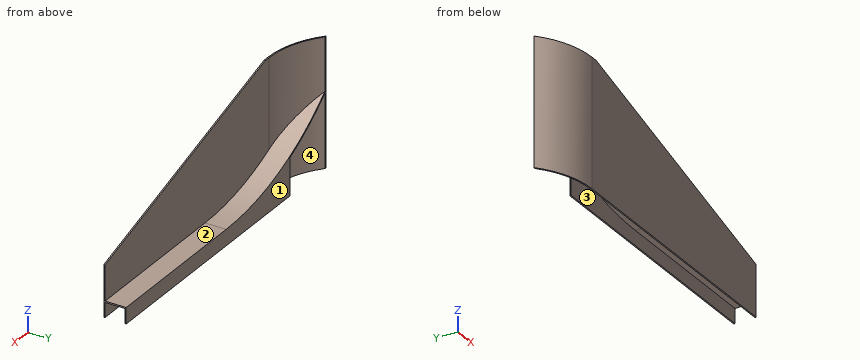
Autodesk Inventor part; units mm, degrees
ref_plane "YZ Plane" through (0, 0, 0) normal (1, 0, 0) x (0, 1, 0)
ref_plane "XZ Plane" through (0, 0, 0) normal (0, 1, 0) x (-1, 0, 0)
ref_plane "XY Plane" through (0, 0, 0) normal (0, 0, 1) x (1, 0, 0)
sketch "スケッチ1" plane through (0, 0, 0) normal (0, 1, 0) x (-1, 0, 0)
  line L0 (250, 100) -> (-250, 100)
  line L1 (-250, 100) -> (-250, -100)
  line L2 (-250, -100) -> (250, -100)
  line L3 (250, -100) -> (250, 100)
  point P0 (0, 0)
  dimension "d2" = 250
  dimension "d3" = 500
  dimension "d4" = 100
  dimension "d5" = 200
extrude "押し出し1" add sketch "スケッチ1" along normal blind 35
sketch "スケッチ2" plane through (-250, 0, 100) normal (0, 0, 1) x (1, 0, 0)
  line L0 (0, 35) -> (500, 35)
  line L1 (0, 0) -> (500, 0)
  arc A0 (0, 35) -> (90, 0) centre (90, 133.2143) ccw
  line L2 (0, 0) -> (0, 35)
  point P0 (250, 0)
  dimension "d8" = 90
extrude "押し出し2" cut sketch "スケッチ2" against normal through all
sketch "スケッチ5" plane through (-160, 0, 100) normal (0, 0, 1) x (1, 0, 0)
  arc A0 (-90, 35) -> (0, 0) centre (0, 133.2143) ccw
  line L0 (0, 0) -> (410, 0)
  arc A1 (-87.0123, 35) -> (0, 2) centre (0, 133.2143) ccw
  line L1 (0, 2) -> (54.4195, 2)
  line L2 (54.4195, 2) -> (410, 2)
  line L3 (-90, 35) -> (410, 35)
  line L4 (410, 0) -> (410, 35)
  point P0 (160, 0)
  point P1 (40, 35)
  dimension "d20" = 2
extrude "押し出し5" cut sketch "スケッチ5" against normal through all contours L3 L4 L2 L1 A1
sketch "スケッチ8" plane through (-160, 2, 100) normal (0, 1, 0) x (1, 0, 0)
  line L0 (410, 175) -> (160, 175)
  line L1 (410, 200) -> (410, 0)
  line L2 (0, 200) -> (410, 200)
  arc A0 (160, 175) -> (-90, 80) centre (160, -201.4474) ccw
  line L3 (-90, 200) -> (-90, 0)
  line L4 (-87.0123, 200) -> (0, 200)
  line L5 (-87.0123, 200) -> (-90, 200)
  line L6 (410, 177) -> (160, 177)
  arc A1 (160, 177) -> (-90, 82.6695) centre (160, -201.4474) ccw
  line L7 (410, 175) -> (410, 177)
  line L8 (410, 0) -> (410, 200)
  line L9 (-90, 82.6695) -> (-90, 80)
  point P0 (160, 100)
  dimension "d35" = 25
  dimension "d36" = 120
  dimension "d37" = 250
  dimension "d38" = 2
extrude "押し出し7" add sketch "スケッチ8" along normal up to surface (33 mm away) contours L0 A0 L3 A1 L6 L1
delete faces "面を削除1" heal yes whole lump no faces at (-239.2435, 9.8792, 10.8013) (-250, 24, 18.2203) (-242.947, 2, 13.2909) (-239.2361, 9.8796, 8.2094)
sketch "スケッチ9" plane through (0, 35, -75) normal (0, 1, 0) x (1, 0, 0)
  line L0 (250, 25) -> (250, 2)
  line L1 (0, 2) -> (250, 2)
  line L2 (250, 25) -> (250, 2)
  line L3 (-160, 25) -> (250, 25)
  line L4 (-160, -33.4861) -> (-160, 25)
  arc A0 (0, 2) -> (-160, -33.4861) centre (0, -376.4474) ccw
  point P0 (0, -75)
extrude "押し出し8" add sketch "スケッチ9" against normal blind 2
sketch "スケッチ10" plane through (-160, 2, 100) normal (0, 1, 0) x (1, 0, 0)
  line L0 (410, 175) -> (410, 0)
  line L1 (410, 0) -> (0, 0)
  line L2 (410, 0) -> (410, 200)
  line L3 (410, 120) -> (10, 0)
  line L4 (0, 0) -> (410, 0)
  point P0 (160, 100)
  dimension "d43" = 400
  dimension "d44" = 120
extrude "押し出し9" cut sketch "スケッチ10" against normal through all
properties part number "endplate_ver2"
Work out the finished part from the listing and answer in its coordinate system (mm). Face numbers are marked on the shaded views. A direction names the side the tool comes from. Coordinates: 2 decimals unless noted, no trailing zeros. Loops run counter-clockwise (first coordinate to the right, second up) from the corner with the lowest first, then second, coordinate; pieces in that order, holes last. Notation, with made-up numbers: M 11,16 L 28,16 A20 ccw 28,34 Z; hole C 10,-6.75 d1. An arc over 180 degrees is marked long. Use CSV: the item, a comma, the result in double quotes. Start each with the question number.
(1) Find section B-B, the plane y = 20. Give the vertices of the cut face in (x, z), then the cut area to 3 significant figures.
(2) Given pin 1 Ø2 at (y, z) = (27, 2) entering from -X; pin 2 Ø4 at (x, z) = (-164.5, -26) entering from +Y; pin 3 Ø8 at (x, y) = (-123, 29.5) entering from +Z, each flat-ended and moving along its own axis, determine where each tip first touches the part or whether it passes through.
(3) For the marked faces 1, 2, 3 and 4, determine the directions among +Z, -Z, +X, -X, +Y, -Y from which every point of the face is accessible in a straight line to the end or side of a thin tool.
(4) Find section D-D, the plane z = 30. Give the vertices of the cut face in (x, y).
(5) Find section A-A, the plane x = 138.5. Give the vertices of the cut face in (y, z), then the cut area to 3 significant figures.
(6) Consider line 1 (Y direction, x = 212, z = -87.5); line 2 (Y direction, x = -146, z = -30); line 3 (Z direction, x = 5, y = 13). Determine where each line is inside the solid, lowest interval first.
Recorded:
1,outline,"M -230.2,-100 L -226.33,-100 L -226.33,-1.86 A378.45 ccw 0,-77 L 250,-77 L 250,-75 L 0,-75 A376.45 cw -226.33,0.64 L -226.33,100 L -230.2,100 Z"
1,area,"1,760 mm^2"
2,pin 1,"stops at x = -241.71"
2,pin 2,"stops at y = 2.16"
2,pin 3,"stops at z = -52.93"
3,face 1,"+Z, -Z, +X, -X, +Y"
3,face 2,"+Z, +X, +Y"
3,face 3,"-Z"
3,face 4,"-Z, +Y"
4,outline,"M -250,35 A133.21 ccw -160,0 L 83.33,0 L 83.33,2 L -160,2 A131.21 cw -247.01,35 Z"
5,outline,"M 0,-100 L 2,-100 L 2,-77 L 33,-77 L 33,-100 L 35,-100 L 35,-75 L 2,-75 L 2,13.45 L 0,13.45 Z"
5,area,"339 mm^2"
6,line 1,"y = 0 to 2, 33 to 35"
6,line 2,"y = 0 to 2"
6,line 3,"z = -77 to -75"
